Part model, mm, in its own coordinate system. A direction names the side the tool comes from. Coordinates: 2 decimals unless noted, no trailing zeros. Loops run counter-clockwise (first coordinate to the right, second up) from the corner with the lowest first, then second, coordinate; pieces in that order, holes last. Notation, with made-up numbers: (-36, 3) -> (5, 3) arc R28 ccw to (5, 23) -> close; hole circle Ø9 at (16, 44). An arc over 180 degrees is marked (long way). One line per item, written item: value. Start each with the question number.
from build123d import *

# Parameters (mm, degrees)
SKETCH1_W           = 419.1
SKETCH1_H           = 333.375
BOSS_EXTRUDE1_DEPTH = 60.325
SKETCH2_W           = 139.7
SKETCH2_H           = 50.8
CUT_EXTRUDE1_DEPTH  = 61.325
CHAMFER1_SIZE       = 50.8
CHAMFER1_SIZE2      = 13.611818976
FILLET1_R           = 12.7
SKETCH3_W           = 139.7
SKETCH3_H           = 56.403006085
CUT_EXTRUDE2_DEPTH  = 12.7
SKETCH4_W           = 139.7
SKETCH4_H           = 56.128435861
CUT_EXTRUDE3_DEPTH  = 12.7
SKETCH5_OUTSIDE_W   = 528.882
SKETCH5_OUTSIDE_H   = 443.156
SKETCH5_OUTSIDE_W_2 = 200.025
SKETCH5_OUTSIDE_H_2 = 333.375
CUT_EXTRUDE4_DEPTH  = 61.325


with BuildPart() as part:
    # Sketch1 → Boss-Extrude1 (new body)
    with BuildSketch(Plane(origin=(0, 0, 0), x_dir=(1, 0, 0), z_dir=(0, 1, 0))):
        Rectangle(SKETCH1_W, SKETCH1_H)
    extrude(amount=BOSS_EXTRUDE1_DEPTH)

    # Sketch2 → Cut-Extrude1 (cut, through all)
    with BuildSketch(Plane(origin=(0, 60.325, 0), x_dir=(1, 0, 0), z_dir=(0, 1, 0))):
        with Locations((0, -115.8875)):
            Rectangle(SKETCH2_W, SKETCH2_H)
        Polygon((-69.85, -166.6875), (-69.85, -157.1625), (-32.169017961, -166.6875), align=None)
        Polygon((32.169017961, -166.6875), (69.85, -166.6875), (69.85, -157.1625), align=None)
    extrude(amount=-CUT_EXTRUDE1_DEPTH, mode=Mode.SUBTRACT)

    # Chamfer1
    chamfer1_edges = [part.edges().sort_by_distance(p)[0] for p in [
        (69.85, 30.1625, 141.2875),
        (-69.85, 30.1625, 141.2875),
    ]]
    chamfer1_side = [part.faces().sort_by_distance(p)[0] for p in [
        (0, 30.1625, 141.2875),
    ]]
    chamfer(chamfer1_edges, length=CHAMFER1_SIZE, length2=CHAMFER1_SIZE2, reference=chamfer1_side[0])

    # Fillet1
    fillet1_edges = [part.edges().sort_by_distance(p)[0] for p in [
        (69.85, 30.1625, 90.4875),
        (-69.85, 30.1625, 90.4875),
        (-32.169017961, 30.1625, 166.6875),
        (32.169017961, 30.1625, 166.6875),
        (69.85, 30.1625, 127.675681024),
        (-19.05, 30.1625, 141.2875),
        (19.05, 30.1625, 141.2875),
        (-69.85, 30.1625, 127.675681024),
    ]]
    fillet(fillet1_edges, radius=FILLET1_R)

    # Sketch3 → Cut-Extrude2 (cut)
    with BuildSketch(Plane(origin=(0, 60.325, 0), x_dir=(1, 0, 0), z_dir=(0, 1, 0))):
        with Locations((0, -138.485996957)):
            Rectangle(SKETCH3_W, SKETCH3_H)
    extrude(amount=-CUT_EXTRUDE2_DEPTH, mode=Mode.SUBTRACT)

    # Sketch4 → Cut-Extrude3 (cut)
    with BuildSketch(Plane.XZ):
        with Locations((0, 138.623282069)):
            Rectangle(SKETCH4_W, SKETCH4_H)
    extrude(amount=-CUT_EXTRUDE3_DEPTH, mode=Mode.SUBTRACT)

    # Sketch5 outside → Cut-Extrude4 (cut, through all)
    with BuildSketch(Plane(origin=(0, 60.325, 0), x_dir=(1, 0, 0), z_dir=(0, 1, 0))):
        Rectangle(SKETCH5_OUTSIDE_W, SKETCH5_OUTSIDE_H)
        Rectangle(SKETCH5_OUTSIDE_W_2, SKETCH5_OUTSIDE_H_2, mode=Mode.SUBTRACT)
    extrude(amount=-CUT_EXTRUDE4_DEPTH, mode=Mode.SUBTRACT)


solid = part.part
1) Slice it at A-A (y = 36). Give the cut face in (x, z).
2) Tool access for faces 4 (the flat face through (-69.85, 30, 113)), 5 (the flat face through (-1, 47.625, 147)), 6 (the flat face through (52.029, 30.407, 161.667)), 7 (the flat face through (-1, 12.7, 148)), 8 (the cylindrical face through (66.23, 29.74, 94.31)): list every direction of +Z, -Z, +X, -X, +Y, -Y with a clear straight run to the whole face (end or side of a thin tool).
3) Pull direction X, two halves, no side cores. Call faces 1 (the flat face through (-1, 31, 90.488)), 2 (the flat face through (-100.012, 31, 2)), 3 (the flat face through (-1, 30, -166.688)): +X half, -X half, draft (parallel to the pull), parting line (faces both ways), or undercut.
4) Slice it at C-C (y = 6). Give the cut face in (x, z), then the cut area to 3 significant figures.
5) Probe line 1 (X direction, y = 49, z = 135); line 2 (Z direction, x = 12, y = 46); line 3 (Z direction, x = 34, y = 31). List the from-to ranges inside material, lowest first. Write a range as from..to.
6) Pin check, flat tip, straight feed: pin 1 Ø24.5 at (x, z) = (16.5, 148) entering from -Y. Stop position of the tip, or through.
Check sheet entries:
1. outline: (-100.01, -166.69) -> (100.01, -166.69) -> (100.01, 166.69) -> (69.85, 166.69) -> (69.85, 157.16) -> (33.7, 166.3) arc R12.7 ccw to (30.59, 166.69) -> (-30.59, 166.69) arc R12.7 ccw to (-33.7, 166.3) -> (-69.85, 157.16) -> (-69.85, 166.69) -> (-100.01, 166.69) -> close; hole (-69.85, 103.19) arc R12.7 ccw to (-57.15, 90.49) -> (57.15, 90.49) arc R12.7 ccw to (69.85, 103.19) -> (69.85, 117.93) arc R12.7 ccw to (60.44, 130.2) -> (20.67, 140.85) arc R12.7 ccw to (17.38, 141.29) -> (-17.38, 141.29) arc R12.7 ccw to (-20.67, 140.85) -> (-60.44, 130.2) arc R12.7 ccw to (-69.85, 117.93) -> close
2. face 4: none
2. face 5: +Z, +Y
2. face 6: +Z, +Y, -Y
2. face 7: +Z, -Y
2. face 8: +Y, -Y
3. face 1: undercut
3. face 2: -X half
3. face 3: draft
4. outline: (-100.01, -166.69) -> (100.01, -166.69) -> (100.01, 166.69) -> (69.85, 166.69) -> (69.85, 103.19) arc R12.7 cw to (57.15, 90.49) -> (-57.15, 90.49) arc R12.7 cw to (-69.85, 103.19) -> (-69.85, 166.69) -> (-100.01, 166.69) -> close
4. area: 56,100 mm^2
5. line 1: x = -100.01..-69.85, 69.85..100.01
5. line 2: z = -166.69..90.49, 141.29..166.69
5. line 3: z = -166.69..90.49, 137.28..166.22
6. pin 1: stops at y = 12.7
